Part model, mm, in its own coordinate system. A direction names the side the tool comes from. Give positions to 0.01 mm unless a question says otherwise; leave off trailing zeros. Write each loop counter-clockwise with the first axis right and the second up, starting at its lowest first coordinate (ties: lowest second). Pieces come first, ordered by that corner, then holes.
from build123d import *

# Parameters (mm, degrees)
RESSALTO_EXTRUS_O1_DEPTH = 139.86
RESSALTO_EXTRUS_O2_DEPTH = 139.86
ESBO_O3_W                = 34.02
ESBO_O3_H                = 95.34
RESSALTO_EXTRUS_O3_DEPTH = 9.24
ESBO_O4_R                = 4.5
CORTE_EXTRUS_O1_DEPTH    = 9.24
RESSALTO_EXTRUS_O4_DEPTH = 34.02
ESBO_O7_W                = 34.02
ESBO_O7_H                = 95.34
RESSALTO_EXTRUS_O5_DEPTH = 9.24
ESBO_O8_R                = 4.5
CORTE_EXTRUS_O3_DEPTH    = 9.24
ESBO_O9_R                = 11.13
CORTE_EXTRUS_O4_DEPTH    = 7.14
RESSALTO_EXTRUS_O6_DEPTH = 34.02
ESBO_O12_R               = 11.13
CORTE_EXTRUS_O5_DEPTH    = 7.14


with BuildPart() as part:
    # Esboço1 → Ressalto-extrusão1 (new body)
    with BuildSketch(Plane.XY):
        Polygon((44.1, -30.03), (49.98, -30.03), (49.98, 30.03), (-49.98, 30.03), (-49.98, -30.03), (-44.1, -30.03), (-44.1, 24.15), (44.1, 24.15), align=None)
    extrude(amount=RESSALTO_EXTRUS_O1_DEPTH)

    # Esboço2 → Ressalto-extrusão2 (add)
    with BuildSketch(Plane.XY.offset(139.86)):
        Polygon((-44.1, 24.15), (-44.1, 14.07), (-34.02, 24.15), align=None)
        Polygon((44.1, 24.15), (44.1, 14.07), (34.02, 24.15), align=None)
    extrude(amount=-RESSALTO_EXTRUS_O2_DEPTH)

    # Esboço3 → Ressalto-extrusão3 (add)
    with BuildSketch(Plane.XY.offset(139.86)):
        with Locations((0, 77.7)):
            Rectangle(ESBO_O3_W, ESBO_O3_H)
    extrude(amount=-RESSALTO_EXTRUS_O3_DEPTH)

    # Esboço4 → Corte-extrusão1 (cut)
    with BuildSketch(Plane.XY.offset(139.86)):
        with Locations((0, 112.35)):
            Circle(ESBO_O4_R)
    extrude(amount=-CORTE_EXTRUS_O1_DEPTH, mode=Mode.SUBTRACT)

    # Esboço6 → Ressalto-extrusão4 (add)
    with BuildSketch(Plane(origin=(17.01, 0, 0), x_dir=(0, 0, -1), z_dir=(1, 0, 0))):
        Polygon((-130.62, 50.19), (-130.62, 30.03), (-110.46, 30.03), align=None)
    extrude(amount=-RESSALTO_EXTRUS_O4_DEPTH)

    # Esboço7 → Ressalto-extrusão5 (add)
    with BuildSketch(Plane(origin=(0, 0, 0), x_dir=(-1, 0, 0), z_dir=(0, 0, -1))):
        with Locations((0, 77.7)):
            Rectangle(ESBO_O7_W, ESBO_O7_H)
    extrude(amount=-RESSALTO_EXTRUS_O5_DEPTH)

    # Esboço8 → Corte-extrusão3 (cut)
    with BuildSketch(Plane(origin=(0, 0, 0), x_dir=(-1, 0, 0), z_dir=(0, 0, -1))):
        with Locations((0, 113.108647766)):
            Circle(ESBO_O8_R)
    extrude(amount=-CORTE_EXTRUS_O3_DEPTH, mode=Mode.SUBTRACT)

    # Esboço9 → Corte-extrusão4 (cut)
    with BuildSketch(Plane(origin=(0, 0, 0), x_dir=(-1, 0, 0), z_dir=(0, 0, -1))):
        with Locations((0, 113.108647766)):
            Circle(ESBO_O9_R)
    extrude(amount=-CORTE_EXTRUS_O4_DEPTH, mode=Mode.SUBTRACT)

    # Esboço10 → Ressalto-extrusão6 (add)
    with BuildSketch(Plane(origin=(17.01, 0, 0), x_dir=(0, 0, -1), z_dir=(1, 0, 0))):
        Polygon((-9.24, 30.03), (-9.24, 50.19), (-29.4, 30.03), align=None)
    extrude(amount=-RESSALTO_EXTRUS_O6_DEPTH)

    # Esboço12 → Corte-extrusão5 (cut)
    with BuildSketch(Plane(origin=(0, 0, 130.62), x_dir=(-1, 0, 0), z_dir=(0, 0, -1))):
        with Locations((0, 112.35)):
            Circle(ESBO_O12_R)
    extrude(amount=-CORTE_EXTRUS_O5_DEPTH, mode=Mode.SUBTRACT)


solid = part.part
1) Saw through at A-A (x = 0). Write the cut outline in (y, z), and give its area (3 significant figures).
Check result:
outline: (24.15, 0) - (101.98, 0) - (101.98, 7.14) - (108.61, 7.14) - (108.61, 9.24) - (50.19, 9.24) - (30.03, 29.4) - (30.03, 110.46) - (50.19, 130.62) - (101.22, 130.62) - (101.22, 137.76) - (107.85, 137.76) - (107.85, 139.86) - (24.15, 139.86) - close; (116.85, 137.76) - (123.48, 137.76) - (123.48, 130.62) - (125.37, 130.62) - (125.37, 139.86) - (116.85, 139.86) - close; (117.61, 7.14) - (124.24, 7.14) - (124.24, 0) - (125.37, 0) - (125.37, 9.24) - (117.61, 9.24) - close
area: 2,640 mm2
2) Saw through at C-C (z = 70). Write the cut outline in (x, y).
Check result:
outline: (-49.98, -30.03) - (-44.1, -30.03) - (-44.1, 14.07) - (-34.02, 24.15) - (34.02, 24.15) - (44.1, 14.07) - (44.1, -30.03) - (49.98, -30.03) - (49.98, 30.03) - (-49.98, 30.03) - close
3) Saw through at B-B (y = 84). Write the cut outline in (x, z).
Check result:
outline: (-17.01, 0) - (17.01, 0) - (17.01, 9.24) - (-17.01, 9.24) - close; (-17.01, 130.62) - (17.01, 130.62) - (17.01, 139.86) - (-17.01, 139.86) - close
4) Saw through at D-D (x = 14). Write the cut outline in (y, z), and give its area (3 significant figures).
Check result:
outline: (24.15, 0) - (125.37, 0) - (125.37, 9.24) - (50.19, 9.24) - (30.03, 29.4) - (30.03, 110.46) - (50.19, 130.62) - (125.37, 130.62) - (125.37, 139.86) - (24.15, 139.86) - close
area: 2,990 mm2
5) Drill centre lines: L1, parallel to Y at x = 0, z = 135; L2, parallel to Y at x = 0, z = 8.45; L3, parallel to X at y = 4, z = 117. Where is each one in solid material? Low to high.
Check result:
L1: y = 24.15 to 101.22, 123.48 to 125.37
L2: y = 24.15 to 108.61, 117.61 to 125.37
L3: x = -49.98 to -44.1, 44.1 to 49.98
6) Mould opens along Y. For faces 1 (the flat face through (0, 125.37, 5)), 2 (the flat face through (-5, 113, 7.14)), 3 (the cylindrical face through (0.59, 117.57, 8.18)), 4 (the flat face through (0, 80, 130.62)) say: +Y half, -Y half, draft (parallel to the pull), parting line (faces both ways), or undercut.
Check result:
face 1: +Y half
face 2: undercut
face 3: undercut
face 4: draft
7) 3-axis set-ups, long thin cutter, end or side, ignore diameter. For faces 5 (the flat face through (17.01, 68, 5)), 6 (the flat face through (44.1, -8, 69)), 7 (the flat face through (0, 88, 9.24)), 8 (the flat face through (1, 30.03, 69)), 9 (the flat face through (-17.01, 68, 135)): which of +Z, -Z, +X, -X, +Y, -Y reach the whole face in a straight line?
Check result:
face 5: +Z, -Z, +X, +Y
face 6: +Z, -Z, -Y
face 7: +X, -X, +Y
face 8: +Y
face 9: +Z, -Z, -X, +Y
8) Flat gauge pins, fed straight in: P1, Ø1.5, axis at x = 3.5, z = 40.5, coming from the +Y side; P2, Ø9, axis at y = 81, z = 16, coming from the +X side; P3, Ø13.5, axis at x = 0, y = 112.35, coming from the -Z side; P4, Ø12, axis at x = 19.5, z = 16.5, coming from the +Y side. Where does each tip first touch, or does it go through?
Check result:
P1: stops at y = 30.03
P2: passes through
P3: stops at z = 7.14
P4: stops at y = 48.39
